Source: three-view drawing plus pictorial views. Frame: mm from the lowest corner of the part. Give positions to 0.01 mm unless a question says otherwise; leave off trailing zeros. Write each loop counter-clockwise with the first axis right and the second up, starting at its lowest first coordinate (ties: lowest second). Pieces come first, ordered by that corner, then holes.
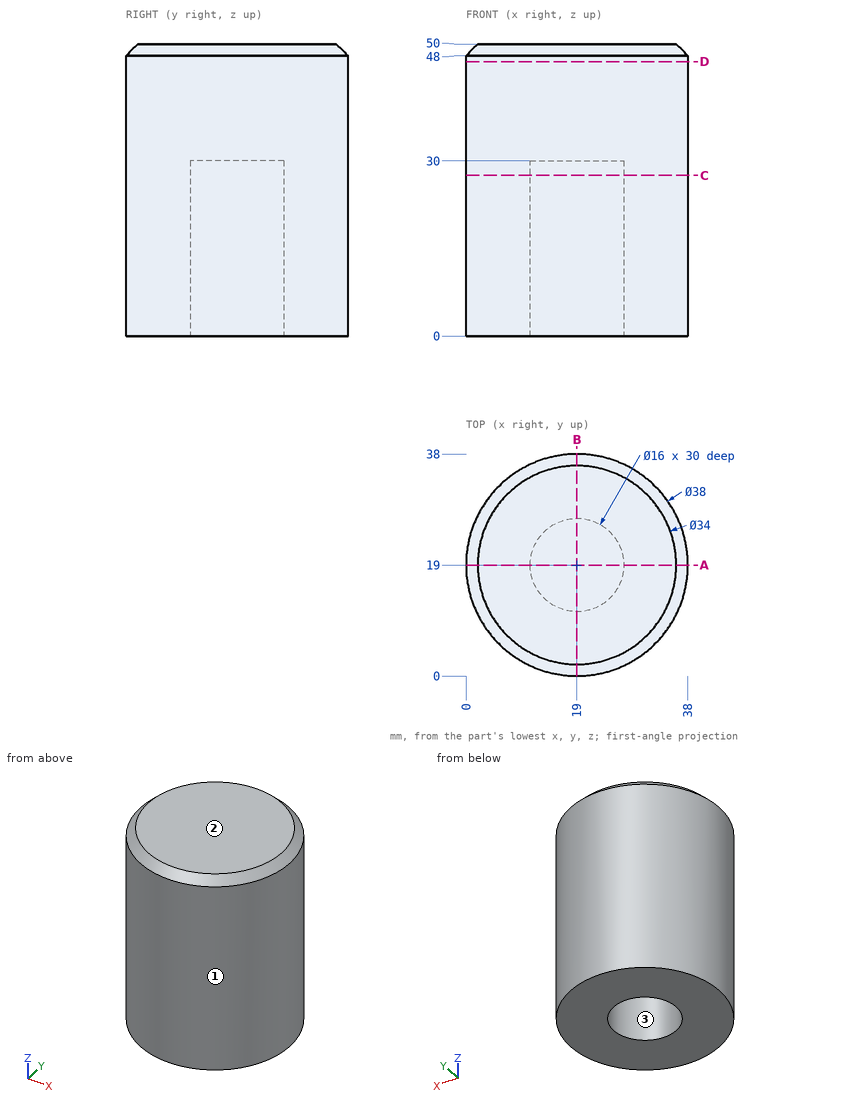
Q1. Pin query (flat end, axial travel): P1, Ø8, axis at y = 21, z = 39.5, coming from the -X side; P2, Ø5, axis at y = 27.5, z = 18, coming from the +X side; P3, Ø1.5, axis at x = 26.5, z = 39, coming from the +Y side; P4, Ø10, axis at x = 15, z = 7.5, coming from the +Y side. Return the tip coordinate at first contact, or that it passes through.
Filled sheet:
P1: stops at x = 0
P2: stops at x = 37.03
P3: stops at y = 36.76
P4: stops at y = 38
Q2. Ray query, line 1 along Y through (x, z) = (19, 22); line 2 along Z through (x, y) = (12, 22.5); line 3 along X through (y, z) = (13, 7). Return the intervals inside material, ascending.
Filled sheet:
line 1: y = 0 to 11, 27 to 38
line 2: z = 30 to 50
line 3: x = 0.97 to 13.71, 24.29 to 37.03
Q3. Section C-C on z = 27.5. Output: boundary loops of the cut face in (x, y).
Filled sheet:
outline: circle Ø38 at (19, 19); hole circle Ø16 at (19, 19)
Q4. Section A-A on y = 19. Output: boundary loops of the cut face in (x, z).
Filled sheet:
outline: (0, 0) - (11, 0) - (11, 30) - (27, 30) - (27, 0) - (38, 0) - (38, 48) - (36, 50) - (2, 50) - (0, 48) - close
Q5. Section D-D on z = 47. Output: boundary loops of the cut face in (x, y).
Filled sheet:
outline: circle Ø38 at (19, 19)
Q6. Pull-direction query (X, two-part tool) for the marked faces 1, 2 and 3; classes: released by +X, released by -X, zero draft, split by the parting line, or undercut.
Filled sheet:
face 1: split by the parting line
face 2: zero draft
face 3: undercut
